```python
from build123d import *

# Parameters (mm, degrees)
SKETCH1_R           = 4
BOSS_EXTRUDE1_DEPTH = 10
SKETCH2_R           = 2.5
CUT_EXTRUDE1_DEPTH  = 8
SKETCH3_R           = 2.5
CUT_EXTRUDE2_DEPTH  = 8


with BuildPart() as part:
    # Sketch1 → Boss-Extrude1 (new body)
    with BuildSketch(Plane.XY):
        with BuildLine():
            Line((0, 0), (0, 31))
            ThreePointArc((0, 31), (2.928932188, 38.071067812), (10, 41))
            Line((10, 41), (50.004448763, 41))
            ThreePointArc((50.004448763, 41), (57.075516575, 38.071067812), (60.004448763, 31))
            Line((60.004448763, 31), (60.004448763, 0))
            Line((60.004448763, 0), (50.004448763, 0))
            Line((50.004448763, 0), (46.002224382, 4.002224382))
            Line((46.002224382, 4.002224382), (46.002224382, 17))
            Line((46.002224382, 17), (14.002224382, 17))
            Line((14.002224382, 17), (14.002224382, 4.002224382))
            Line((14.002224382, 4.002224382), (10, 0))
            Line((10, 0), (0, 0))
        make_face()
        with Locations((30.002224382, 31)):
            Circle(SKETCH1_R, mode=Mode.SUBTRACT)
    extrude(amount=BOSS_EXTRUDE1_DEPTH)

    # Sketch2 → Cut-Extrude1 (cut)
    with BuildSketch(Plane.XZ):
        with Locations(Location((55.004448763, 5, 0), (0, 0, 270))):
            Circle(SKETCH2_R)
    extrude(amount=-CUT_EXTRUDE1_DEPTH, mode=Mode.SUBTRACT)

    # Sketch3 → Cut-Extrude2 (cut)
    with BuildSketch(Plane.XZ):
        with Locations(Location((5, 5, 0), (0, 0, 270))):
            Circle(SKETCH3_R)
    extrude(amount=-CUT_EXTRUDE2_DEPTH, mode=Mode.SUBTRACT)


solid = part.part
```
The listing builds one solid part. Answer for the finished solid, in the listing's coordinates (mm). A direction names the side the tool comes from. Coordinates: 2 decimals unless noted, no trailing zeros. Write each loop counter-clockwise with the first axis right and the second up, starting at its lowest first coordinate (ties: lowest second). Pieces come first, ordered by that corner, then holes.
Q1. The mould has two halves that part along Z. Classify faces 1 (the cylindrical face through (2.85, 37.99, 4.93)), 2 (the cylindrical face through (5.751, 3.944, 2.615)), 3 (the flat face through (30, 25, 0)): released by +Z, released by -Z, zero draft, split by the parting line, or undercut.
Returned:
face 1: zero draft
face 2: undercut
face 3: released by -Z
Q2. Find the intervals of material crossed by line 1 along X through (y, z) = (5.5, 5); line 2 along X through (y, z) = (12, 7); line 3 along X through (y, z) = (3.5, 4.75), in increasing order.
Returned:
line 1: x = 0 to 2.5, 7.5 to 14, 46 to 52.5, 57.5 to 60
line 2: x = 0 to 14, 46 to 60
line 3: x = 0 to 2.51, 7.49 to 13.5, 46.5 to 52.52, 57.49 to 60
Q3. Given P1, Ø1, axis at x = 43, z = 7.5, coming from the -Y side; P2, Ø9, axis at x = 30, y = 31, coming from the +Z side; P3, Ø2.5, axis at x = 55, z = 6, coming from the -Y side; P4, Ø1, axis at x = 13.5, z = 5, coming from the -Y side, each flat-ended and moving along its own axis, determine where each tip first touches the part or whether it passes through.
Returned:
P1: stops at y = 17
P2: stops at z = 10
P3: stops at y = 8
P4: stops at y = 3
Q4. Section B-B, the plane z = 5 is taken. Write down the section's boundary in (x, y), then the cut area to 3 significant figures.
Returned:
outline: (0, 0) - (2.5, 0) - (2.5, 8) - (7.5, 8) - (7.5, 0) - (10, 0) - (14, 4) - (14, 17) - (46, 17) - (46, 4) - (50, 0) - (52.5, 0) - (52.5, 8) - (57.5, 8) - (57.5, 0) - (60, 0) - (60, 31) arc R10 ccw to (50, 41) - (10, 41) arc R10 ccw to (0, 31) - close; hole circle Ø8 at (30, 31)
area: 1,730 mm2
Q5. Section A-A, the plane y = 14.5 is taken. Write down the section's boundary in (x, z).
Returned:
outline: (0, 0) - (14, 0) - (14, 10) - (0, 10) - close; (46, 0) - (60, 0) - (60, 10) - (46, 10) - close
Q6. Section C-C, the plane y = 6 is taken. Write down the section's boundary in (x, z).
Returned:
outline: (0, 0) - (14, 0) - (14, 10) - (0, 10) - close; (46, 0) - (60, 0) - (60, 10) - (46, 10) - close; hole circle Ø5 at (5, 5); hole circle Ø5 at (55, 5)
Q7. Section D-D, the plane z = 8.75 is taken. Write down the section's boundary in (x, y).
Returned:
outline: (0, 0) - (10, 0) - (14, 4) - (14, 17) - (46, 17) - (46, 4) - (50, 0) - (60, 0) - (60, 31) arc R10 ccw to (50, 41) - (10, 41) arc R10 ccw to (0, 31) - close; hole circle Ø8 at (30, 31)
Q8. Which of the six approach directions +Z, -Z, +X, -X, +Y, -Y give full straight-line access (tool end or side, diameter ignored) to faces 4 (the flat face through (12, 2, 5)), 5 (the flat face through (30, 25, 10)), 6 (the flat face through (5, 8, 5))?
Returned:
face 4: +Z, -Z, -Y
face 5: +Z, +X, -X, +Y, -Y
face 6: -Y
